from build123d import *

# Parameters (mm, degrees)
F0_W     = 60
F0_H     = 60
F0_R     = 1.6112939769
F1_DEPTH = 3
F2_SIZE  = 5


with BuildPart() as f1:
    # F0 (on Top) → F1 (new body)
    with BuildSketch(Plane.XY):
        with Locations((24.9740350166, -9.1694972429)):
            Rectangle(F0_W, F0_H)
        with BuildLine():
            Line((3.2622774597, -15.6086981297), (16.5645107627, -10.5752451345))
            Line((16.5645107627, -10.5752451345), (16.5645107627, -15.204295516))
            add(Edge.make_bspline(
                [(16.5645107627, -19.1635359079), (14.8224645411, -19.6451143125), (11.7558446548, -20.4928632954), (6.1547440409, -20.5448956868), (11.8429032498, -17.426394245), (14.8983947786, -15.9884085963), (16.5645107627, -15.204295516)],
                knots=[0, 0, 0, 0, 0.2743421374, 0.4829395706, 0.7180543169, 1, 1, 1, 1], degree=3))
            Line((16.5645107627, -19.1635359079), (16.5645107627, -22.8168163449))
            add(Edge.make_bspline(
                [(16.5645107627, -22.8168163449), (14.4725531382, -23.2798512694), (10.0419202377, -24.2605297243), (0.6256088462, -22.3279022421), (0.2660082773, -16.7243281021), (2.3214114275, -15.9590199071), (3.2622774597, -15.6086981297)],
                knots=[0, 0, 0, 0, 0.2846115058, 0.6027890272, 0.8181756645, 1, 1, 1, 1], degree=3))
        make_face(mode=Mode.SUBTRACT)
        with Locations((45.2274344862, -25.2090897411)):
            Circle(F0_R, mode=Mode.SUBTRACT)
        with BuildLine():
            Line((27.5594554842, -19.4526854903), (27.5594554842, -14.2551343888))
            Line((27.5594554842, -14.2551343888), (34.5340929925, -13.0454646423))
            add(Edge.make_bspline(
                [(34.5340929925, -13.0454646423), (37.2063908175, -12.6439263534), (42.3024714088, -11.8781915384), (53.478633217, -18.6523955934), (37.6371992304, -23.7025636039), (27.378866449, -26.9728675485)],
                knots=[0, 0, 0, 0, 0.2798359986, 0.5336481539, 1, 1, 1, 1], degree=3))
            Line((27.378866449, -26.9728675485), (27.378866449, -22.2297701985))
            add(Edge.make_bspline(
                [(34.2456139624, -16.9829949737), (35.640261338, -16.5033856088), (37.9383903882, -15.7130752885), (40.0731287249, -15.8571844549), (40.2704488484, -17.8896647841), (33.0974326396, -20.3045464891), (27.378866449, -22.2297701985)],
                knots=[0, 0, 0, 0, 0.2546068482, 0.4195464779, 0.5372432196, 1, 1, 1, 1], degree=3))
            Line((34.2456139624, -16.9829949737), (27.5594554842, -19.4526854903))
        make_face(mode=Mode.SUBTRACT)
        with BuildLine():
            Line((18.2588193566, -24.9153450131), (18.2588193566, 11.3608455285))
            add(Edge.make_bspline(
                [(32.6563753188, -11.9998930022), (33.6693549813, -11.8025701643), (36.1962896301, -11.3103372651), (38.2049388483, -4.0554139358), (37.4316089742, 7.077116303), (25.3393667705, 9.7788562356), (18.2588193566, 11.3608455285)],
                knots=[0, 0, 0, 0, 0.1494558255, 0.3728259491, 0.6327616062, 1, 1, 1, 1], degree=3))
            Line((32.6563753188, -11.9998930022), (28.2806474715, -10.3766387329))
            Line((28.2806474715, -10.3766387329), (28.2806474715, 2.468238119))
            Line((28.2806474715, 2.468238119), (28.2100718468, 3.597458126))
            Line((28.2100718468, 3.597458126), (27.1867176699, 4.6208149288))
            Line((27.1867176699, 4.6208149288), (26.1633582413, 3.597458126))
            Line((26.1633582413, 3.597458126), (26.1633582413, 1.7624760512))
            Line((26.1633582413, 1.7624760512), (26.1633582413, -27.1737873554))
            Line((26.1633582413, -27.1737873554), (25.1752920449, -27.1737873554))
            Line((25.1752920449, -27.1737873554), (18.2588193566, -24.9153450131))
        make_face(mode=Mode.SUBTRACT)
    extrude(amount=F1_DEPTH)

    # F2
    f2_edges = [f1.edges().sort_by_distance(p)[0] for p in [
        (-5.025965, 20.830503, 1.5),
        (-5.025965, -39.169497, 1.5),
        (54.974035, -39.169497, 1.5),
        (54.974035, 20.830503, 1.5),
    ]]
    chamfer(f2_edges, length=F2_SIZE)


solid = f1.part
Geometry check sheet. Reference: the model listing, model coordinates, mm. A direction names the side the tool comes from. Round coordinates to 2 decimals unless told otherwise and drop trailing zeros.
Item 1: Thickness scan on line 1 (X direction, y = -2, z = 1.5); line 2 (X direction, y = -9.5, z = 2.8); line 3 (Y direction, x = 40, z = 2.25). Record the ranges inside material, lowest first.
Item 2: Mould release check, pull along X, two halves, no side actions. Record for faces 3 (the flat face through (-2.491, -36.704, 1.479)), 4 (the flat face through (16.565, -13, 1)), 5 (the flat face through (25, 20.831, 1)), 6 (the flat face through (30.5, -11.2, 1.5)): pulls with the +X half, pulls with the -X half, needs draft (parallel to the pull), parting line crosses it, or undercut.
Item 3: Access from +Z, -Z, +X, -X, +Y, -Y to the whole of each face (thin tool, end or side, straight path). Record for faces 1 (the flat face through (-5.026, -10, 1)), 2 (the flat face through (31, -13.66, 1.48)).
Item 4: Cross-section at A-A on y = -26. Count the separate pieces of the cut face and the enclosed holes in it, then the cut area to 3 significant figures.
Answer sheet:
1. line 1: x = -5.03 to 18.26, 26.16 to 28.28, 37.79 to 54.97
1. line 2: x = -5.03 to 18.26, 26.16 to 28.28, 36.37 to 54.97
1. line 3: y = -39.17 to -22.69, -16.78 to -16.23, -12.6 to 20.83
2. face 3: pulls with the -X half
2. face 4: undercut
2. face 5: needs draft
2. face 6: undercut
3. face 1: +Z, -Z, -X, +Y, -Y
3. face 2: +Z, -Z
4. separate pieces: 4
4. enclosed holes: 0
4. area: 149 mm2
